Autodesk Inventor part; units mm, degrees
ref_plane "YZ Plane" through (0, 0, 0) normal (1, 0, 0) x (0, 1, 0)
ref_plane "XZ Plane" through (0, 0, 0) normal (0, 1, 0) x (-1, 0, 0)
ref_plane "XY Plane" through (0, 0, 0) normal (0, 0, 1) x (1, 0, 0)
sketch "Sketch1" plane through (0, 0, 0) normal (0, 1, 0) x (-1, 0, 0)
  line L0 (0, 0) -> (0, -1219.2)
  line L1 (0, 0) -> (88.9, 0)
  line L2 (88.9, 0) -> (88.9, -1219.2)
  line L3 (88.9, -1219.2) -> (0, -1219.2)
  line L4 (0, 0) -> (0, 1219.2) construction
  line L5 (0, 1219.2) -> (1219.2, 1219.2) construction
  line L6 (0, 1219.2) -> (0, 3657.6) construction
  line L7 (0, 3657.6) -> (0, 4876.8) construction
  line L8 (0, 4876.8) -> (0, 6096) construction
  line L9 (0, -1219.2) -> (2438.4, -1219.2) construction
  line L10 (0, 6096) -> (2438.4, 6096) construction
  line L11 (2438.4, 6096) -> (2438.4, -1219.2) construction
  line L12 (0, 3657.6) -> (0, 3352.8) construction
  line L13 (0, 3352.8) -> (2438.4, 3352.8) construction
  line L14 (2438.4, 3352.8) -> (1219.2, 3352.8)
  line L15 (1219.2, 3352.8) -> (1219.2, 3263.9)
  line L16 (1219.2, 3263.9) -> (2438.4, 3263.9)
  line L17 (2438.4, 3263.9) -> (2438.4, 3352.8)
  line L18 (0, 6096) -> (862.1046, 6958.1046)
  line L19 (862.1046, 6958.1046) -> (924.9664, 6895.2428)
  line L20 (924.9664, 6895.2428) -> (62.8618, 6033.1382)
  line L21 (62.8618, 6033.1382) -> (0, 6096)
  line L22 (0, 4876.8) -> (1219.2, 4876.8) construction
  line L23 (1219.2, 4876.8) -> (2081.3046, 5738.9046)
  line L24 (1219.2, 1219.2) -> (2081.3046, 357.0954)
  line L25 (2081.3046, 357.0954) -> (2018.4428, 294.2336)
  line L26 (2018.4428, 294.2336) -> (1156.3382, 1156.3382)
  line L27 (1156.3382, 1156.3382) -> (1219.2, 1219.2)
  line L28 (2018.4428, 294.2336) -> (88.9, -1219.2)
  line L29 (2081.3046, 357.0954) -> (2144.1664, 419.9572)
  line L30 (2144.1664, 419.9572) -> (1282.0618, 1282.0618)
  line L31 (1282.0618, 1282.0618) -> (1219.2, 1219.2)
  line L32 (2438.4, 3352.8) -> (2438.4, 3441.7)
  line L33 (2438.4, 3441.7) -> (1219.2, 3441.7)
  line L34 (1219.2, 3441.7) -> (1219.2, 3352.8)
  line L35 (1156.3382, 4939.6618) -> (1282.0618, 4813.9382)
  line L36 (2018.4428, 5801.7664) -> (2144.1664, 5676.0428)
  line L37 (1282.0618, 4813.9382) -> (2144.1664, 5676.0428)
  line L38 (2018.4428, 5801.7664) -> (1156.3382, 4939.6618)
  line L39 (2018.4428, 5801.7664) -> (924.9664, 6895.2428)
  line L40 (62.8618, 6033.1382) -> (1156.3382, 4939.6618)
  line L41 (1233.6206, 4168.8855) -> (1267.6412, 4086.7527)
  line L42 (1263.7078, 2313.9849) -> (1230.0006, 2231.7229)
  arc A0 (862.1046, 6958.1046) -> (0, 6096) centre (431.0523, 6527.0523) ccw
  line L43 (1246.8542, 2272.8539) -> (2375.0183, 1810.583)
  line L44 (2391.8719, 1851.7139) -> (2358.1646, 1769.452)
  line L45 (2391.8719, 1851.7139) -> (1263.7078, 2313.9849)
  line L46 (1230.0006, 2231.7229) -> (2358.1646, 1769.452)
  line L47 (1230.0006, 2231.7229) -> (1219.2, 3263.9)
  line L48 (2144.1664, 419.9572) -> (2391.8719, 1851.7139)
  line L49 (2391.8719, 1851.7139) -> (2438.4, 3263.9)
  line L50 (1219.2, 3441.7) -> (1233.6206, 4168.8855)
  line L51 (1250.6309, 4127.8191) -> (2377.0248, 4594.3867)
  line L52 (2360.0145, 4635.4532) -> (2394.0351, 4553.3203)
  line L53 (2394.0351, 4553.3203) -> (1267.6412, 4086.7527)
  line L54 (2360.0145, 4635.4532) -> (1233.6206, 4168.8855)
  line L55 (2394.0351, 4553.3203) -> (2144.1664, 5676.0428)
  line L56 (2438.4, 3441.7) -> (2394.0351, 4553.3203)
  line L57 (2144.1664, 5676.0428) -> (2057.3895, 5656.7301)
  line L58 (2394.0351, 4553.3203) -> (2305.2058, 4549.7751)
  line L59 (2394.0351, 4553.3203) -> (2307.2582, 4534.0076)
  line L60 (2307.2582, 4534.0076) -> (2057.3895, 5656.7301)
  line L61 (2438.4, 3441.7) -> (2349.5707, 3438.1548)
  line L62 (2349.5707, 3438.1548) -> (2305.2058, 4549.7751)
  line L63 (1219.2, 3441.7) -> (1308.0825, 3439.9374)
  line L64 (1233.6206, 4168.8855) -> (1322.5031, 4167.1229)
  line L65 (1322.5031, 4167.1229) -> (1308.0825, 3439.9374)
  line L66 (2018.4428, 5801.7664) -> (1955.581, 5738.9046)
  line L67 (1955.581, 5738.9046) -> (862.1046, 6832.381)
  line L68 (924.9664, 6895.2428) -> (862.1046, 6832.381)
  line L69 (62.8618, 6033.1382) -> (125.7236, 6096)
  line L70 (62.8618, 6033.1382) -> (125.7236, 6096)
  line L71 (125.7236, 6096) -> (1219.2, 5002.5236)
  line L72 (1156.3382, 1156.3382) -> (0, 0)
  line L73 (0, 0) -> (62.8618, -62.8618)
  line L74 (1156.3382, 1156.3382) -> (1219.2, 1093.4764)
  line L75 (1219.2, 1093.4764) -> (62.8618, -62.8618)
  line L76 (2018.4428, 294.2336) -> (1963.5776, 364.1837)
  line L77 (88.9, -1219.2) -> (34.0348, -1149.2499)
  line L78 (34.0348, -1149.2499) -> (1963.5776, 364.1837)
  line L79 (2144.1664, 419.9572) -> (2056.5677, 435.1125)
  line L80 (2391.8719, 1851.7139) -> (2304.2732, 1866.8692)
  line L81 (2391.8719, 1851.7139) -> (2303.0201, 1854.6414)
  line L82 (2304.2732, 1866.8692) -> (2056.5677, 435.1125)
  line L83 (1230.0006, 2231.7229) -> (1318.8957, 2232.6531)
  line L84 (1219.2, 3263.9) -> (1308.0951, 3264.8302)
  line L85 (1308.0951, 3264.8302) -> (1318.8957, 2232.6531)
  line L86 (2438.4, 3263.9) -> (2349.5482, 3266.8275)
  line L87 (2349.5482, 3266.8275) -> (2303.0201, 1854.6414)
  line L88 (88.9, 0) -> (125.7236, 0)
  line L89 (1233.6206, 4168.8855) -> (1219.2, 4876.8)
  line L90 (1233.6206, 4168.8855) -> (1322.5022, 4170.6961)
  line L91 (1219.2, 4876.8) -> (1308.0816, 4878.6106)
  line L92 (1308.0816, 4878.6106) -> (1322.5022, 4170.6961)
  line L93 (1282.0618, 4813.9382) -> (1309.9674, 4786.0326)
  line L94 (1267.6412, 4086.7527) -> (1318.4756, 3964.0275)
  line L95 (2360.0145, 4635.4532) -> (2374.4273, 4641.4231)
  line L96 (1230.0006, 2231.7229) -> (1219.2, 1219.2)
  line L97 (1230.0006, 2231.7229) -> (1318.8955, 2230.7747)
  line L98 (1219.2, 1219.2) -> (1308.0949, 1218.2518)
  line L99 (1308.0949, 1218.2518) -> (1318.8955, 2230.7747)
  line L100 (1282.0618, 1282.0618) -> (1309.0636, 1309.0636)
  point P0 (1770.957, 2057.4547)
  point P1 (1955.1236, 357.5528)
  point P2 (88.9, -1106.2164)
  dimension "d0" = 1219.2
  dimension "d2" = 1219.2
  dimension "d3" = 1219.2
  dimension "d16" = 2438.4
  dimension "d17" = 1219.2
  dimension "d18" = 1219.2
  dimension "d20" = 2438.4
  dimension "d21" = 304.8
  dimension "d22" = 1219.2
  dimension "d23" = 88.9
  dimension "d24" = 1219.2
  dimension "d25" = 45
  dimension "d26" = 88.9
  dimension "d27" = 1219.2
  dimension "d28" = 1219.2
  dimension "d29" = 1219.2
  dimension "d31" = 1219.2
  dimension "d32" = 88.9
  dimension "d33" = 88.9
  dimension "d34" = 88.9
  dimension "d35" = 177.8
  dimension "d36" = 177.8
  dimension "d38" = 88.9
  dimension "d39" = 88.9
  dimension "d43" = 1219.2
  dimension "d44" = 88.9
  dimension "d45" = 1219.2
  dimension "d46" = 88.9
  dimension "d47" = 88.9
  dimension "d48" = 88.9
  dimension "d49" = 88.9
  dimension "d50" = 88.9
  dimension "d51" = 88.9
  dimension "d54" = 88.9
  dimension "d55" = 88.9
  dimension "d57" = 88.9
  dimension "d58" = 88.9
  dimension "d59" = 88.9
  dimension "d60" = 88.9
  dimension "d61" = 88.9
  dimension "d64" = 88.9
  dimension "d65" = 88.9
  dimension "d66" = 88.9
  dimension "d69" = 88.9
  dimension "d70" = 88.9
  dimension "d71" = 88.9
  dimension "d72" = 88.9
extrude "Extrusion1" add sketch "Sketch1" along normal blind 38.1 contours L72 L26 L75 L88 L1
properties part number "S_2x4x64.382"
For this review, take the finished solid that the model builds, in its own axes (mm). Coordinates: 2 decimals unless noted, no trailing zeros. Order: outer loops, then holes, each group sorted by start corner. A loop starts at its lowest first (then second) coordinate and runs counter-clockwise, first axis right, second up. Notation, with made-up numbers: (63, -9) - (105, -9) arc R8 ccw to (105, -1) - close; hole circle Ø11 at (85.25, 56.25). An arc over 180 degrees is marked (long way). Answer as CSV lines item,"result". Start each with the question number.
1) Insertion check: P1, Ø10, axis at x = -1089.5, y = 25, coming from the -Z side; P2, Ø4, axis at x = -722.5, y = 8, coming from the +Z side; P3, Ø12, axis at y = 21.5, z = 495, coming from the +X side. Each pin has a flat end and moves straight along its axis. Give the tip position at first contact, or say it passes through.
2) Add section A-A (x = -102.5). State the section outline as (y, z) points.
3) To check wall thickness, follow line 1 along Z through (x, y) = (-732.5, 25.5); line 2 along Z through (x, y) = (-477, 4); line 3 along X through (y, z) = (13, 135). State the ranges of each line that lie inside material, in increasing order. Write a range as [from, to].
4) Add section B-B (y = 25). State the section outline as (x, z) points, then the cut area to 3 significant figures.
Result:
1,P1,"z = 958.78"
1,P2,"z = 724.5"
1,P3,"x = -489"
2,outline,"(0, 0) - (38.1, 0) - (38.1, 102.5) - (0, 102.5) - close"
3,line 1,"[606.78, 732.5]"
3,line 2,"[351.28, 477]"
3,line 3,"[-260.72, -135]"
4,outline,"(-1219.2, 1093.48) - (-125.72, 0) - (0, 0) - (-1156.34, 1156.34) - close"
4,area,"141,000 mm^2"
